from build123d import *

# Parameters (mm, degrees)
F0_R     = 1.55
F1_DEPTH = 9.9
F2_W     = 8.4
F2_H     = 11.5120084733
F2_W_2   = 12.9466587678
F2_H_2   = 19.0824847668
F3_DEPTH = 25
F4_R     = 4.99999
F5_SIZE  = 4


# Not quite as in the source:
# - a fillet or chamfer is up to 0.001 mm smaller than in the source, because OpenCascade refuses the exact size
# - a feature names something its author has since deleted; it is built from what else it names


with BuildPart() as f1:
    # F0 (on Right) → F1 (new body, symmetric)
    with BuildSketch(Plane.YZ):
        with BuildLine():
            Line((-5, 25.5), (-5, -20))
            Line((-5, -20), (5, -20))
            Line((5, -20), (5, 25.5))
            Line((5, 25.5), (1.55, 25.5))
            ThreePointArc((1.55, 25.5), (0, 23.95), (-1.55, 25.5))
            Line((-1.55, 25.5), (-5, 25.5))
        make_face()
        with Locations((0, -15.5)):
            Circle(F0_R, mode=Mode.SUBTRACT)
        with Locations((0, 15.5)):
            Circle(F0_R, mode=Mode.SUBTRACT)
        with BuildLine():
            ThreePointArc((5, 25.5), (0, 30.5), (-5, 25.5))
            Line((-5, 25.5), (-1.55, 25.5))
            ThreePointArc((-1.55, 25.5), (0, 27.05), (1.55, 25.5))
            Line((1.55, 25.5), (5, 25.5))
        make_face()
    extrude(amount=F1_DEPTH, both=True)

    # F2 (on face) → F3 (cut)
    with BuildSketch(Plane.XZ.offset(5)):
        with Locations((0, 25.5)):
            Rectangle(F2_W, F2_H)
        Rectangle(F2_W_2, F2_H_2)
    extrude(amount=-F3_DEPTH, mode=Mode.SUBTRACT)

    # F4 (radius 5 in the source; OpenCascade refuses exactly that, so slightly less here)
    f4_edges = [f1.edges().sort_by_distance(p)[0] for p in [
        (0, -5, 19.743996),
        (0, 5, 19.743996),
    ]]
    fillet(f4_edges, radius=F4_R)

    # F5
    f5_edges = [f1.edges().sort_by_distance(p)[0] for p in [
        (6.473329, 0, 9.541242),
        (-6.473329, 0, 9.541242),
    ]]
    chamfer(f5_edges, length=F5_SIZE)


solid = f1.part
Here's how the part is built. I have some questions about the finished solid (model axes, mm). A direction names the side the tool comes from. Coordinates: 2 decimals unless noted, no trailing zeros. Order: outer loops, then holes, each group sorted by start corner. A loop starts at its lowest first (then second) coordinate and runs counter-clockwise, first axis right, second up. Notation, with made-up numbers: (75, 17.25) -> (88, 17.25) arc R26 ccw to (88, 32.25) -> close; hole circle Ø1 at (44, -14). An arc over 180 degrees is marked (long way). Answer in a Markdown table with one row per item.
(1) On a 3-axis mill with a long thin cutter (end or side, diameter ignored), from which of +Z, -Z, +X, -X, +Y, -Y can I reach the whole of each face in a straight line? I mean faces 4 (the face through (-7, 0.1, 30.5)), 5 (the face through (-4.501, -0.07, 7.513)). Say none if no direction works.
Answer key:
| item | result |
|---|---|
| face 4 | +Z, +X, -X |
| face 5 | +Y, -Y |
(2) I want a section at D-D on y = 4.25. List the corners of the cut face in (x, z) for me, then the cut area to 3 significant figures.
Answer key:
| item | result |
|---|---|
| outline | (-9.9, -20) -> (9.9, -20) -> (9.9, 28.13) -> (4.2, 28.13) -> (4.2, 17.38) -> (-4.2, 17.38) -> (-4.2, 28.13) -> (-9.9, 28.13) -> close; hole (-6.47, -9.54) -> (6.47, -9.54) -> (6.47, 5.54) -> (2.47, 9.54) -> (-2.47, 9.54) -> (-6.47, 5.54) -> close |
| area | 632 mm^2 |
(3) I want a section at B-B on z = -15.5. List the corners of the cut face in (x, y) for me, then the cut area to 3 significant figures.
Answer key:
| item | result |
|---|---|
| outline | (-9.9, -5) -> (9.9, -5) -> (9.9, -1.55) -> (-9.9, -1.55) -> close; (-9.9, 1.55) -> (9.9, 1.55) -> (9.9, 5) -> (-9.9, 5) -> close |
| area | 137 mm^2 |
(4) Thinking about a two-plate mould opening in Y: for faces 1 (the face through (0, 0, -9.541)), 2 (the face through (-0.139, -0.202, -13.963)), 3 (the face through (0.059, -3.574, 18.24)), which applies, +Y half, -Y half, draft (parallel to the pull), parting line (faces both ways), or undercut?
Answer key:
| item | result |
|---|---|
| face 1 | draft |
| face 2 | undercut |
| face 3 | -Y half |
(5) I want a section at C-C on x = -4.75. List the corners of the cut face in (y, z) for me.
Answer key:
| item | result |
|---|---|
| outline | (-5, -20) -> (5, -20) -> (5, -9.54) -> (-5, -9.54) -> close; (-5, 7.26) -> (5, 7.26) -> (5, 25.5) arc R5 ccw to (-5, 25.5) -> close; hole circle Ø3.1 at (0, -15.5); hole circle Ø3.1 at (0, 15.5); hole circle Ø3.1 at (0, 25.5) |
(6) Please list where these lines run through material, in increasing order: probe 1 along Z at (x, y) = (0.5, 0); probe 2 along Z at (x, y) = (7.95, 0); probe 3 along X at (y, z) = (-0.5, -8).
Answer key:
| item | result |
|---|---|
| probe 1 | -20 to -17.05, -13.95 to -9.54, 9.54 to 13.95, 17.05 to 19.74 |
| probe 2 | -20 to -17.05, -13.95 to 13.95, 17.05 to 23.95, 27.05 to 30.5 |
| probe 3 | -9.9 to -6.47, 6.47 to 9.9 |
(7) I want a section at A-A on x = -0.75. Count the separate pieces of the cut face and the enclosed holes in it, then the cut area to 3 significant figures.
Answer key:
| item | result |
|---|---|
| separate pieces | 2 |
| enclosed holes | 2 |
| area | 181 mm^2 |
